Could you check a few things on this model? Use its own coordinates, in mm. Face numbers are marked on the shaded views. A direction names the side the tool comes from. Coordinates: 2 decimals unless noted, no trailing zeros. Write item = value, one per line. Start each with the question number.
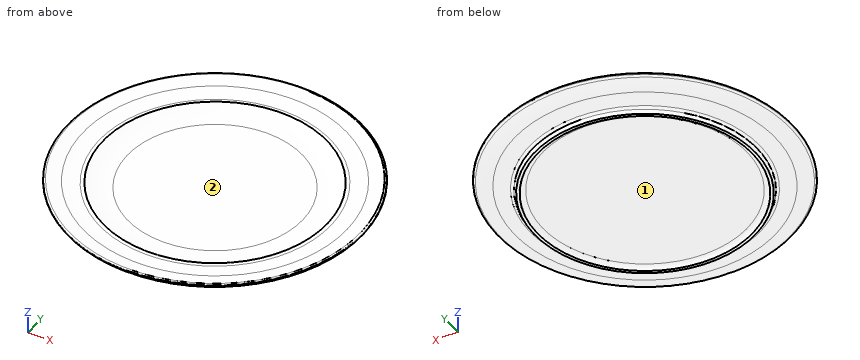
```python
from build123d import *


# Not quite as in the source:
# - a fillet or chamfer that OpenCascade refuses, or shapes differently, is made with other operations: its cross-section is extruded or revolved along the edge and cut away or added


with BuildPart() as f1:
    # F0 (on Front) → F1 (revolve)
    with BuildSketch(Plane.XZ):
        with BuildLine():
            Line((100, 0), (0, 0))
            Line((0, 0), (0, -2.6495179627))
            Line((0, -2.6495179627), (91.3194956564, -2.6495179627))
            ThreePointArc((91.3194956564, -2.6495179627), (94.0684515249, -3.473007262), (95.9119130966, -5.6722213094))
            Line((95.9119130966, -5.6722213094), (95.9628000855, -5.7904100977))
            Line((95.9628000855, -5.7904100977), (98.6674576998, -5.7904100977))
            ThreePointArc((98.6674576998, -5.7904100977), (99.3204777078, -4.1476735329), (100.3251448274, -2.6931418106))
            ThreePointArc((100.3251448274, -2.6931418106), (101.5086125026, -1.71503666), (102.9425561428, -1.1663190089))
            ThreePointArc((102.9425561428, -1.1663190089), (109.6751369936, 0.1797320354), (116.4222210646, 1.4510914916))
            ThreePointArc((116.4222210646, 1.4510914916), (123.2251802907, 3.0758263676), (129.8146396875, 5.4208301008))
            ThreePointArc((129.8146396875, 5.4208301008), (130.7332526352, 5.961479711), (131.4723342657, 6.7295357585))
            ThreePointArc((131.4723342657, 6.7295357585), (131.6712873102, 7.3402645066), (131.4723342657, 7.9509932548))
            ThreePointArc((131.4723342657, 7.9509932548), (130.7405288737, 8.5304559761), (129.8146396875, 8.648969233))
            ThreePointArc((129.8146396875, 8.648969233), (123.6657142098, 7.6457790436), (117.5564303994, 6.4241709188))
            ThreePointArc((117.5564303994, 6.4241709188), (110.44281422, 5.2047996177), (103.2479256392, 4.6356073581))
            ThreePointArc((103.2479256392, 4.6356073581), (101.6107063419, 4.6996452731), (100, 5))
            Line((100, 5), (100, 0))
        make_face()
    revolve(axis=Axis((0, 0, -1.3247589814), (0, 0, -1)))

    # F2: fillet of radius 50 on 1 edges, made by hand

    # F2_s1 → F2_t2 (revolve)
    with BuildSketch(Plane.XZ):
        with BuildLine():
            ThreePointArc((100, 5), (89.3858451698, 1.266028276), (78.2055052823, 0))
            Line((78.2055052823, 0), (78.2055052823, -1))
            Line((78.2055052823, -1), (100, -1))
            Line((100, -1), (101, 0))
            ThreePointArc((101, 0), (101, 2.5), (100.4358898944, 4.1))
            Line((100.4358898944, 4.1), (100, 5))
        make_face()
    revolve(axis=Axis((0, 0, 0), (0, 0, -1)))


solid = f1.part
```
1) For P1, Ø3, axis at x = 51, z = 5.5, coming from the +Y side; P2, Ø8, axis at x = -26.5, z = 6.5, coming from the +Y side; P3, Ø4, axis at x = -57.5, y = 38.5, coming from the +Z side, each with a flat end and sliding along its axis, tell me the tip position at first contact or that it passes through.
2) If I drill on probe 1 along Z at (x, y) = (33, -22.5); probe 2 along X at (y, z) = (-60, -4.75); probe 3 along X at (y, z) = (-38.5, -4.75), over which ranges is the centre line in solid material (lowest first)? Write a range as [from, to].
3) Which directions (+Z, -Z, +X, -X, +Y, -Y) give clear straight access to the entire face, cutting with the end or side of a thin tool? Please do the marked faces 1 and 2.
Reply:
q1.P1 = 121.54
q1.P2 = 129.72
q1.P3 = 0
q2.probe_1 = [-2.65, 0]
q2.probe_2 = [-78.78, -74.16], [74.16, 78.78]
q2.probe_3 = [-91.24, -87.28], [87.28, 91.24]
q3.face_1 = -Z
q3.face_2 = +Z
